Job drawing, mm, ordinate dimensions from the low corner. One solid piece. A direction names the side the tool comes from. Round coordinates to 2 decimals unless told otherwise and drop trailing zeros. Order: outer loops, then holes, each group sorted by start corner. A loop starts at its lowest first (then second) coordinate and runs counter-clockwise, first axis right, second up. Notation, with made-up numbers: (-30, 81) -> (22, 81) arc R10 ccw to (22, 99) -> close; hole circle Ø10 at (-34, 51.5). An arc over 180 degrees is marked (long way). Return JSON: item names as keys, results as strings. Group by question number.
Q1. Mould opens along Z. For the marked faces 4, 5, 6 and 7 say: +Z half, -Z half, draft (parallel to the pull), parting line (faces both ways), or undercut.
Q2. Cut at A-A (y = 60). Write the cut outline in (x, z), then the cut area to 3 significant figures.
Q3. Which spindle directions (+Z, -Z, +X, -X, +Y, -Y) get a long thin tool onto all of the face, cutting with end or side? Do the marked faces 1, 2 and 3. Say none if no direction does.
Q4. Cut at C-C (x = 15). Write the cut outline in (y, z).
Q5. Cut at D-D (z = 18.5). Write the cut outline in (x, y).
Q6. Cut at B-B (z = 10). Write the cut outline in (x, y), then the cut area to 3 significant figures.
Q7. Probe line 1 along Y through (x, z) = (15, 18.65); line 2 along Y through (x, z) = (16.75, 10); line 3 along Y through (x, z) = (5, 12.75). List the from-to ranges inside material, lowest first.
Q8. Flat gauge pins, fed straight in: pin 1 (1.5 mm diameter, centred on y = 17.5, z = 13, fed in from -X); pin 2 (8 mm diameter, centred on y = 80, z = 10, fed in from +X); pin 3 (2.5 mm diameter, centred on x = 5, y = 60, fed in from +Z); pin 4 (1.6 mm diameter, centred on x = 13.5, z = 0.5, fed in from -Y). Where does each tip first touch, or does it go through?
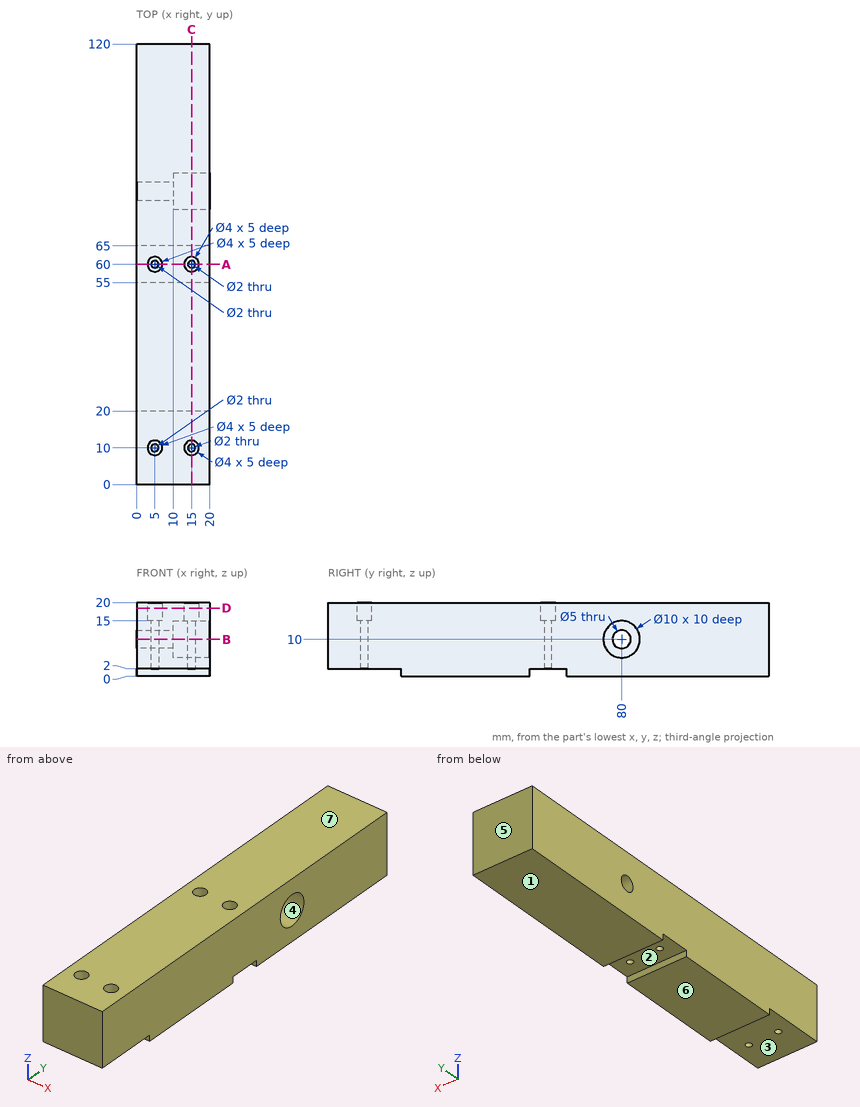
Solution:
{
 "1": {"face 4": "undercut", "face 5": "draft", "face 6": "-Z half", "face 7": "+Z half"},
 "2": {"outline": "(0, 2) -> (4, 2) -> (4, 15) -> (3, 15) -> (3, 20) -> (0, 20) -> close; (6, 2) -> (14, 2) -> (14, 15) -> (13, 15) -> (13, 20) -> (7, 20) -> (7, 15) -> (6, 15) -> close; (16, 2) -> (20, 2) -> (20, 20) -> (17, 20) -> (17, 15) -> (16, 15) -> close", "area": "268 mm²"},
 "3": {"face 1": "-Z, +X, -X, +Y, -Y", "face 2": "-Z, +X, -X", "face 3": "-Z, +X, -X, -Y"},
 "4": {"outline": "(0, 2) -> (9, 2) -> (9, 15) -> (8, 15) -> (8, 20) -> (0, 20) -> close; (11, 2) -> (20, 2) -> (20, 0) -> (55, 0) -> (55, 2) -> (59, 2) -> (59, 15) -> (58, 15) -> (58, 20) -> (12, 20) -> (12, 15) -> (11, 15) -> close; (61, 2) -> (65, 2) -> (65, 0) -> (120, 0) -> (120, 20) -> (62, 20) -> (62, 15) -> (61, 15) -> close; hole circle Ø10 at (80, 10)"},
 "5": {"outline": "(0, 0) -> (20, 0) -> (20, 120) -> (0, 120) -> close; hole circle Ø4 at (5, 10); hole circle Ø4 at (5, 60); hole circle Ø4 at (15, 10); hole circle Ø4 at (15, 60)"},
 "6": {"outline": "(0, 0) -> (20, 0) -> (20, 75) -> (10, 75) -> (10, 77.5) -> (0, 77.5) -> close; (0, 82.5) -> (10, 82.5) -> (10, 85) -> (20, 85) -> (20, 120) -> (0, 120) -> close; hole circle Ø2 at (5, 10); hole circle Ø2 at (5, 60); hole circle Ø2 at (15, 10); hole circle Ø2 at (15, 60)", "area": "2,240 mm²"},
 "7": {"line 1": "y = 0 to 8, 12 to 58, 62 to 120", "line 2": "y = 0 to 75, 85 to 120", "line 3": "y = 0 to 9, 11 to 59, 61 to 120"},
 "8": {"pin 1": "stops at x = 0", "pin 2": "stops at x = 10", "pin 3": "stops at z = 15", "pin 4": "stops at y = 20"}
}
